Verification items for the finished model (mm, model axes). Coordinates: 2 decimals unless noted, no trailing zeros. Loops run counter-clockwise (first coordinate to the right, second up) from the corner with the lowest first, then second, coordinate; pieces in that order, holes last. Notation, with made-up numbers: (47.5, 73) -> (79.5, 73) arc R10 ccw to (79.5, 80) -> close; hole circle Ø10 at (63, 48). An arc over 180 degrees is marked (long way). Write item = value, one per line.
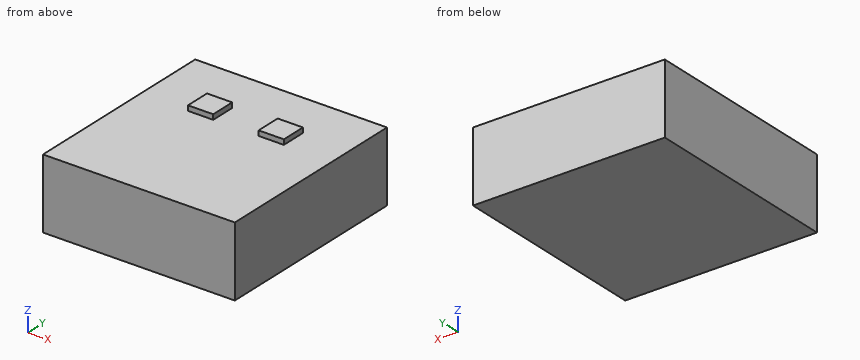
```python
from build123d import *

# Parameters (mm, degrees)
SKETCH_1_W      = 38
SKETCH_1_H      = 40
EXTRUDE_1_DEPTH = 14
SKETCH_2_W      = 5
SKETCH_2_H      = 5
EXTRUDE_2_DEPTH = 1


with BuildPart() as part:
    # 草图1 → 凸台-拉伸1 (new body)
    with BuildSketch(Plane.XY):
        with Locations((19, 20)):
            Rectangle(SKETCH_1_W, SKETCH_1_H)
    extrude(amount=EXTRUDE_1_DEPTH)

    # 草图2 → 凸台-拉伸2 (add)
    with BuildSketch(Plane.XY.offset(14)):
        with Locations((26, 28)):
            Rectangle(SKETCH_2_W, SKETCH_2_H)
        with Locations((12, 28)):
            Rectangle(SKETCH_2_W, SKETCH_2_H)
    extrude(amount=EXTRUDE_2_DEPTH)


solid = part.part
```
1) Sectioned sample at D-D, the plane y = 5.5. Record the cut outline in (x, z).
Ans:
outline = (0, 0) -> (38, 0) -> (38, 14) -> (0, 14) -> close
2) Sectioned sample at C-C, the plane x = 15.5. Record the cut outline in (y, z).
Ans:
outline = (0, 0) -> (40, 0) -> (40, 14) -> (0, 14) -> close
3) Sectioned sample at B-B, the plane x = 24.5. Record the cut outline in (y, z), plus the area to 3 significant figures.
Ans:
outline = (0, 0) -> (40, 0) -> (40, 14) -> (30.5, 14) -> (30.5, 15) -> (25.5, 15) -> (25.5, 14) -> (0, 14) -> close
area = 565 mm2
4) Material ranges on line 1 (Z direction, x = 9, y = 35.5), recorded low to high.
Ans:
line_1 = 0 to 14
5) Sectioned sample at A-A, the plane y = 28.5. Record the cut outline in (x, z).
Ans:
outline = (0, 0) -> (38, 0) -> (38, 14) -> (28.5, 14) -> (28.5, 15) -> (23.5, 15) -> (23.5, 14) -> (14.5, 14) -> (14.5, 15) -> (9.5, 15) -> (9.5, 14) -> (0, 14) -> close
6) Depth check by flat-ended pin: pin 1 Ø1.1 at (y, z) = (27.5, 14.5) entering from -X; pin 2 Ø0.8 at (x, z) = (12.5, 14.5) entering from +Y; pin 3 Ø1 at (x, y) = (6, 10) entering from +Z; pin 4 Ø0.5 at (x, z) = (12, 14.5) entering from -Y. Enter the tip coordinate at first touch or a pass-through.
Ans:
pin_1 = 0
pin_2 = 30.5
pin_3 = 14
pin_4 = 25.5
